Geometry check sheet. Reference: the model listing, model coordinates, mm. Face numbers are marked on the shaded views. Coordinates: 2 decimals unless noted, no trailing zeros. Loops run counter-clockwise (first coordinate to the right, second up) from the corner with the lowest first, then second, coordinate; pieces in that order, holes last.
from build123d import *

# Parameters (mm, degrees)
BASE_SKETCH_R      = 25.4
BASE_SKETCH_R_2    = 13.335
BASE_SKETCH_R_3    = 1.905
BASE_EXTRUDE_DEPTH = 3.175


with BuildPart() as part:
    # Base Sketch → Base Extrude (new body)
    with BuildSketch(Plane.XY):
        Circle(BASE_SKETCH_R)
        Circle(BASE_SKETCH_R_2, mode=Mode.SUBTRACT)
        with Locations((0, 22.225)):
            Circle(BASE_SKETCH_R_3, mode=Mode.SUBTRACT)
        with Locations((19.247414599, 11.1125)):
            Circle(BASE_SKETCH_R_3, mode=Mode.SUBTRACT)
        with Locations((19.247414599, -11.1125)):
            Circle(BASE_SKETCH_R_3, mode=Mode.SUBTRACT)
        with Locations((0, -22.225)):
            Circle(BASE_SKETCH_R_3, mode=Mode.SUBTRACT)
        with Locations((-19.247414599, -11.1125)):
            Circle(BASE_SKETCH_R_3, mode=Mode.SUBTRACT)
        with Locations((-19.247414599, 11.1125)):
            Circle(BASE_SKETCH_R_3, mode=Mode.SUBTRACT)
    extrude(amount=-BASE_EXTRUDE_DEPTH)


solid = part.part
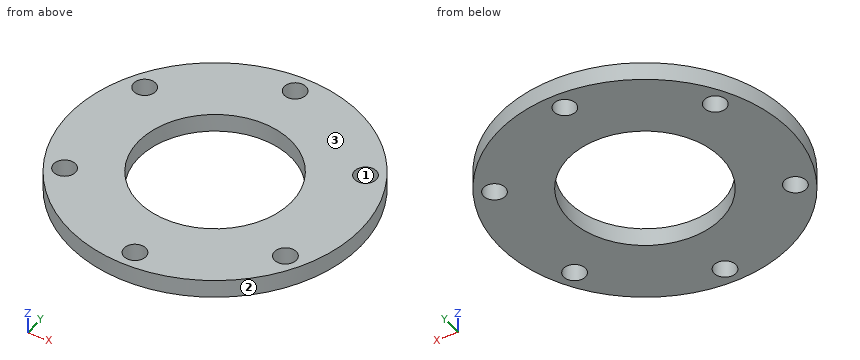
1) Section check D-D on x = 7.5. Record the cut outline in (y, z) (3 decimals).
Data:
outline: (-24.267, -3.175) - (-11.026, -3.175) - (-11.026, 0) - (-24.267, 0) - close; (11.026, -3.175) - (24.267, -3.175) - (24.267, 0) - (11.026, 0) - close
2) Section check A-A on y = 0. Record the cut outline in (x, z) (3 decimals).
Data:
outline: (-25.4, -3.175) - (-13.335, -3.175) - (-13.335, 0) - (-25.4, 0) - close; (13.335, -3.175) - (25.4, -3.175) - (25.4, 0) - (13.335, 0) - close
3) Section check C-C on x = 19. Record the cut outline in (y, z) (3 decimals).
Data:
outline: (-16.857, -3.175) - (-13.001, -3.175) - (-13.001, 0) - (-16.857, 0) - close; (-9.224, -3.175) - (9.224, -3.175) - (9.224, 0) - (-9.224, 0) - close; (13.001, -3.175) - (16.857, -3.175) - (16.857, 0) - (13.001, 0) - close
4) Depth check by flat-ended pin: pin 1 (1 mm diameter, centred on x = -15, z = -3, fed in from -Y); pin 2 (3.5 mm diameter, centred on x = 0, y = 22.225, fed in from -Z); pin 3 (1 mm diameter, centred on x = 4, z = -2, fed in from +Y); pin 4 (4.5 mm diameter, centred on x = 0, y = -22.225, fed in from -Z) (3 decimals). Enter the tip coordinate at first touch or a pass-through.
Data:
pin 1: stops at y = -20.85
pin 2: passes through
pin 3: stops at y = 25.16
pin 4: stops at z = -3.175
5) Material ranges on probe 1 along Y at (x, z) = (0, -0.85) (3 decimals); probe 2 along X at (y, z) = (-10, -2.8); probe 3 along X at (y, z) = (0.5, -1), recorded low to high.
Data:
probe 1: y = -25.4 to -24.13, -20.32 to -13.335, 13.335 to 20.32, 24.13 to 25.4
probe 2: x = -23.35 to -20.79, -17.7 to -8.82, 8.82 to 17.7, 20.79 to 23.35
probe 3: x = -25.4 to -13.33, 13.33 to 25.4
6) Mould release check, pull along X, two halves, no side actions. Record for the marked faces 1, 2 and 3: +X half, -X half, draft (parallel to the pull), parting line (faces both ways), or undercut.
Data:
face 1: undercut
face 2: parting line
face 3: draft
7) Section check B-B on x = 0. Record the cut outline in (y, z) (3 decimals).
Data:
outline: (-25.4, -3.175) - (-24.13, -3.175) - (-24.13, 0) - (-25.4, 0) - close; (-20.32, -3.175) - (-13.335, -3.175) - (-13.335, 0) - (-20.32, 0) - close; (13.335, -3.175) - (20.32, -3.175) - (20.32, 0) - (13.335, 0) - close; (24.13, -3.175) - (25.4, -3.175) - (25.4, 0) - (24.13, 0) - close
